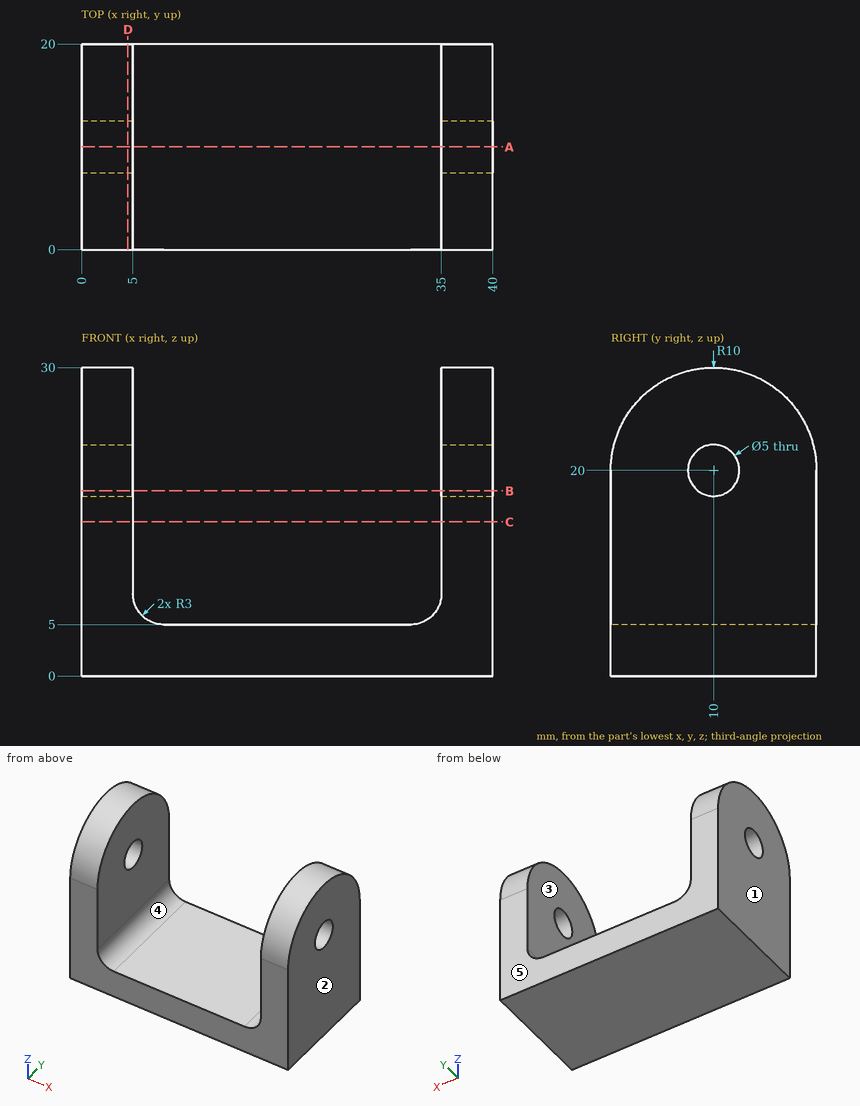
The figure shows three views and two pictorial views of one solid part (mm, origin at its lowest corner). Answer the questions. A direction names the side the tool comes from. Give positions to 0.01 mm unless a question says otherwise; leave off trailing zeros. Order: outer loops, then holes, each group sorted by start corner. A loop starts at its lowest first (then second) coordinate and runs counter-clockwise, first axis right, second up. Notation, with made-up numbers: (-26.5, 85.5) -> (24.5, 85.5) arc R21 ccw to (24.5, 100.5) -> close; hole circle Ø4 at (-7, 5). An arc over 180 degrees is marked (long way). Answer as CSV lines item,"result". Start each with the question number.
Q1. Given pin 1 (10 mm diameter, centred on x = 14.5, y = 13, fed in from +Z); pin 2 (5 mm diameter, centred on y = 6.5, z = 16.5, fed in from -X); pin 3 (4 mm diameter, centred on x = 36, z = 22.5, fed in from -Y); pin 4 (2 mm diameter, centred on x = 7, y = 9.5, fed in from +Z), each flat-ended and moving along its own axis, determine where each tip first touches the part or whether it passes through.
Q2. A cutting plane is placed at A-A (y = 10). Determine the outline of the cut face in (x, z), then the cut area to 3 significant figures.
Q3. Find the intervals of material crossed by L1, parallel to X at y = 7.5, z = 21.5; L2, parallel to Z at x = 38.75, y = 10; L3, parallel to Z at x = 22.5, y = 12.75, in increasing order.
Q4. Determine the mould class of the marked faces 1, 2 and 3 for opening direction X: pulls with the +X half, pulls with the -X half, needs draft (parallel to the pull), parting line crosses it, or undercut.
Q5. A cutting plane is placed at D-D (x = 4.5). Determine the outline of the cut face in (y, z).
Q6. A cutting plane is placed at C-C (z = 15). Determine the outline of the cut face in (x, y), then the cut area to 3 significant figures.
Q7. Which of the six approach directions +Z, -Z, +X, -X, +Y, -Y give full straight-line access (tool end or side, diameter ignored) to the marked faces 4 and 5?
Q8. A cutting plane is placed at B-B (z = 18). Determine the outline of the cut face in (x, y).
Results found:
1,pin 1,"z = 5"
1,pin 2,"x = 0"
1,pin 3,"y = 0.01"
1,pin 4,"z = 5.76"
2,outline,"(0, 0) -> (40, 0) -> (40, 17.5) -> (35, 17.5) -> (35, 8) arc R3 cw to (32, 5) -> (8, 5) arc R3 cw to (5, 8) -> (5, 17.5) -> (0, 17.5) -> close; (0, 22.5) -> (5, 22.5) -> (5, 30) -> (0, 30) -> close; (35, 22.5) -> (40, 22.5) -> (40, 30) -> (35, 30) -> close"
2,area,"404 mm2"
3,L1,"0 to 5, 35 to 40"
3,L2,"0 to 17.5, 22.5 to 30"
3,L3,"0 to 5"
4,face 1,"pulls with the -X half"
4,face 2,"pulls with the +X half"
4,face 3,"undercut"
5,outline,"(0, 0) -> (20, 0) -> (20, 20) arc R10 ccw to (0, 20) -> close; hole circle Ø5 at (10, 20)"
6,outline,"(0, 0) -> (5, 0) -> (5, 20) -> (0, 20) -> close; (35, 0) -> (40, 0) -> (40, 20) -> (35, 20) -> close"
6,area,"200 mm2"
7,face 4,"+Z, +Y, -Y"
7,face 5,"+Z, -Z, +X, -X, +Y"
8,outline,"(0, 0) -> (5, 0) -> (5, 8.5) -> (0, 8.5) -> close; (0, 11.5) -> (5, 11.5) -> (5, 20) -> (0, 20) -> close; (35, 0) -> (40, 0) -> (40, 8.5) -> (35, 8.5) -> close; (35, 11.5) -> (40, 11.5) -> (40, 20) -> (35, 20) -> close"
